Check sheet for the modelled part. Datum: model origin and axes. Units: mm. Coordinates: 2 decimals unless noted, no trailing zeros. Write each loop counter-clockwise with the first axis right and the second up, starting at its lowest first coordinate (ties: lowest second). Pieces come first, ordered by that corner, then holes. Notation, with made-up numbers: (2.25, -39) - (39.25, -39) arc R27 ccw to (39.25, -21) - close; hole circle Ø2 at (26.25, 11.5). An arc over 180 degrees is marked (long way). Write each question's results on one line, items separated by ' | '.
Autodesk Inventor part; units mm, degrees
ref_plane "YZ Plane" through (0, 0, 0) normal (1, 0, 0) x (0, 1, 0)
ref_plane "XZ Plane" through (0, 0, 0) normal (0, 1, 0) x (-1, 0, 0)
ref_plane "XY Plane" through (0, 0, 0) normal (0, 0, 1) x (1, 0, 0)
sketch "Sketch1" plane through (0, 0, 0) normal (0, 1, 0) x (-1, 0, 0)
  line L0 (203.2, 25.4) -> (0, 25.4)
  line L1 (0, 25.4) -> (0, 0)
  line L2 (0, 0) -> (203.2, 0)
  line L3 (203.2, 0) -> (203.2, 25.4)
extrude "Extrusion1" add sketch "Sketch1" along normal blind 2.54
sketch "Sketch2" plane through (0, 2.54, 0) normal (0, 1, 0) x (1, 0, 0)
  circle A0 centre (-12.7, -12.7) radius 6.35
  point P0 (0, 0)
  dimension "d2" = 12.7
sketch "Sketch3" plane through (-203.2, 0, 0) normal (-1, 0, 0) x (0, 0, 1)
  line L0 (25.4, 0) -> (0, 0)
  line L1 (25.4, 0) -> (25.4, 2.54)
  line L2 (0, 2.54) -> (25.4, 2.54)
  line L3 (0, 0) -> (0, 2.54)
extrude "Extrusion2" add sketch "Sketch3" along normal blind 12.7
sketch "Sketch4" plane through (0, 2.54, 0) normal (0, 1, 0) x (1, 0, 0)
  circle A0 centre (-203.2, -12.7) radius 6.35
  point P0 (0, 0)
  dimension "d5" = 12.7
extrude "Extrusion3" cut sketch "Sketch4" against normal blind 2.54
extrude "Extrusion4" cut sketch "Sketch2" against normal blind 2.54
properties part number "4barBar"
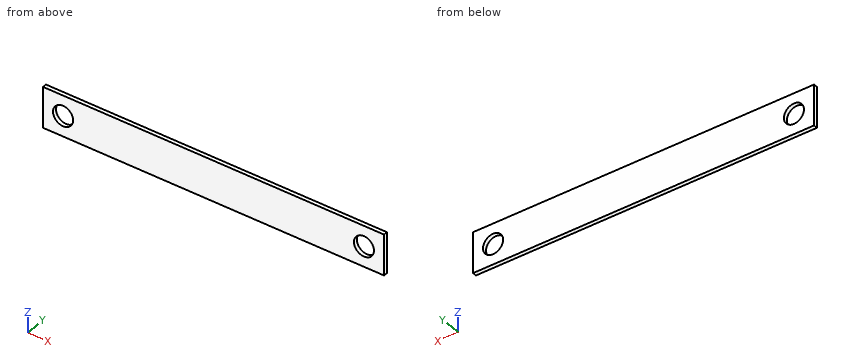
1. Go/stop test with a flat-tipped pin: pin 1 (11.5 mm diameter, centred on x = -203.2, z = 12.7, fed in from -Y). Record where the tip stops, or that it passes through.
Values follow:
pin 1: passes through
2. Sectioned sample at A-A (x = -12.7). Record the cut outline in (y, z), then the cut area to 3 significant figures.
Values follow:
outline: (0, 0) - (2.54, 0) - (2.54, 6.35) - (0, 6.35) - close; (0, 19.05) - (2.54, 19.05) - (2.54, 25.4) - (0, 25.4) - close | area: 32.3 mm^2
3. Material ranges on L1, parallel to X at y = 1.9, z = 12.7; L2, parallel to Z at x = -203.2, y = 1.45; L3, parallel to X at y = 2.1, z = 10, recorded low to high. Write a range as [from, to].
Values follow:
L1: x = [-215.9, -209.55], [-196.85, -19.05], [-6.35, 0] | L2: z = [0, 6.35], [19.05, 25.4] | L3: x = [-215.9, -208.95], [-197.45, -18.45], [-6.95, 0]
4. Sectioned sample at B-B (z = 12.7). Record the cut outline in (x, y), then the cut area to 3 significant figures.
Values follow:
outline: (-215.9, 0) - (-209.55, 0) - (-209.55, 2.54) - (-215.9, 2.54) - close; (-196.85, 0) - (-19.05, 0) - (-19.05, 2.54) - (-196.85, 2.54) - close; (-6.35, 0) - (0, 0) - (0, 2.54) - (-6.35, 2.54) - close | area: 484 mm^2
5. Sectioned sample at C-C (y = 2.05). Record the cut outline in (x, z).
Values follow:
outline: (-215.9, 0) - (0, 0) - (0, 25.4) - (-215.9, 25.4) - close; hole circle Ø12.7 at (-203.2, 12.7); hole circle Ø12.7 at (-12.7, 12.7)
